Design review of the part shown in the three views and the two pictorial views. Dimensions are in mm from the part's minimum x, y and z. Give positions to 0.01 mm unless a question says otherwise; leave off trailing zeros. Order: outer loops, then holes, each group sorted by start corner. A loop starts at its lowest first (then second) coordinate and runs counter-clockwise, first axis right, second up. Notation, with made-up numbers: (17.5, 80.25) -> (72.5, 80.25) arc R13 cw to (72.5, 88.25) -> close; hole circle Ø1 at (-12, 53). An arc over 180 degrees is marked (long way). Answer in a Markdown table with one row per item. Add a question column.
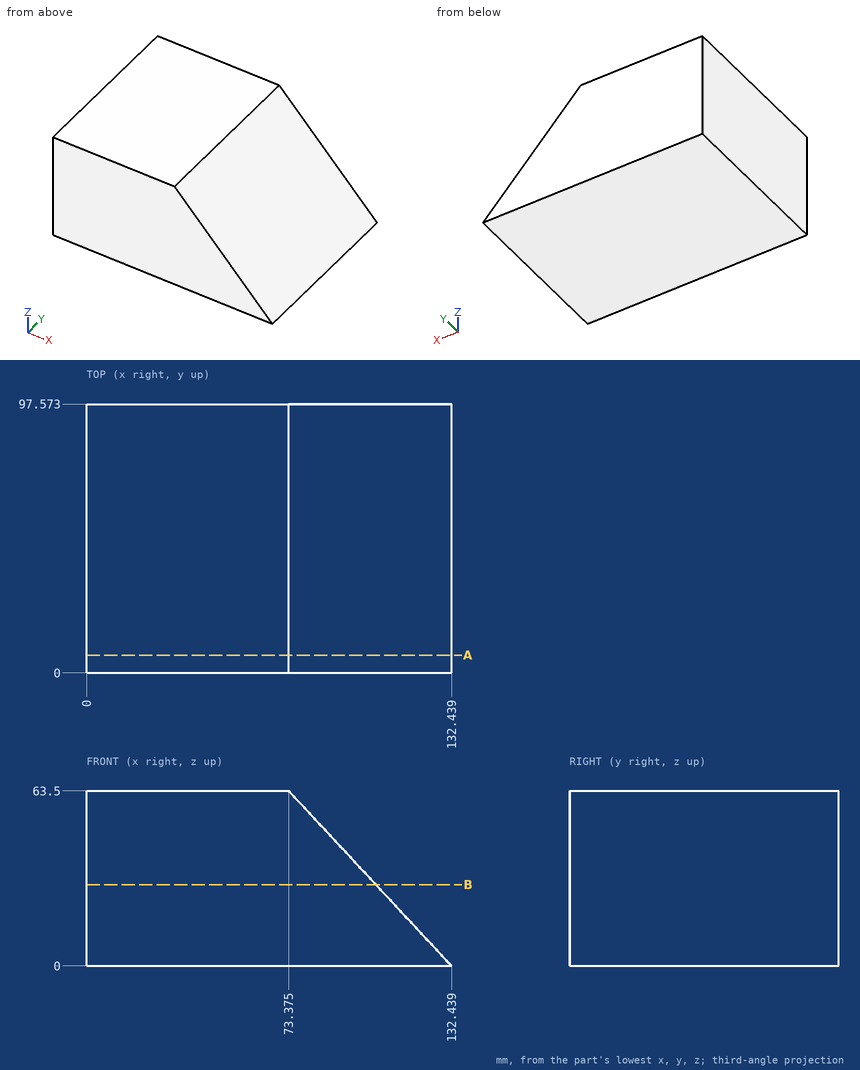
1) Add section B-B, the plane z = 29.5. Write out the cut boundary in (x, y), and give its area (3 significant figures).
2) Clearance check with flat-ended pins moving along their axes: P1, Ø1.5, axis at x = 104.5, y = 10, coming from the +Z side (1 decimal); P2, Ø10, axis at y = 65, z = 45, coming from the +X side. State where each tip first meets the part, or that it passes through.
3) For L1, parallel to X at y = 62.5, z = 60; L2, parallel to Z at x = 90.5, y = 18; L3, parallel to X at y = 19, z = 17.5, list the stretches that pass through material, from the lowest coordinate up.
4) Add section A-A, the plane y = 6.5. Write out the cut boundary in (x, z) (1 decimal).
Verdict:
| question | item | result |
|---|---|---|
| 1 | outline | (0, 0) -> (105, 0) -> (105, 97.57) -> (0, 97.57) -> close |
| 1 | area | 10,200 mm2 |
| 2 | P1 | stops at z = 30.8 |
| 2 | P2 | stops at x = 95.23 |
| 3 | L1 | x = 0 to 76.63 |
| 3 | L2 | z = 0 to 45.09 |
| 3 | L3 | x = 0 to 116.16 |
| 4 | outline | (0, 0) -> (132.4, 0) -> (73.4, 63.5) -> (0, 63.5) -> close |
